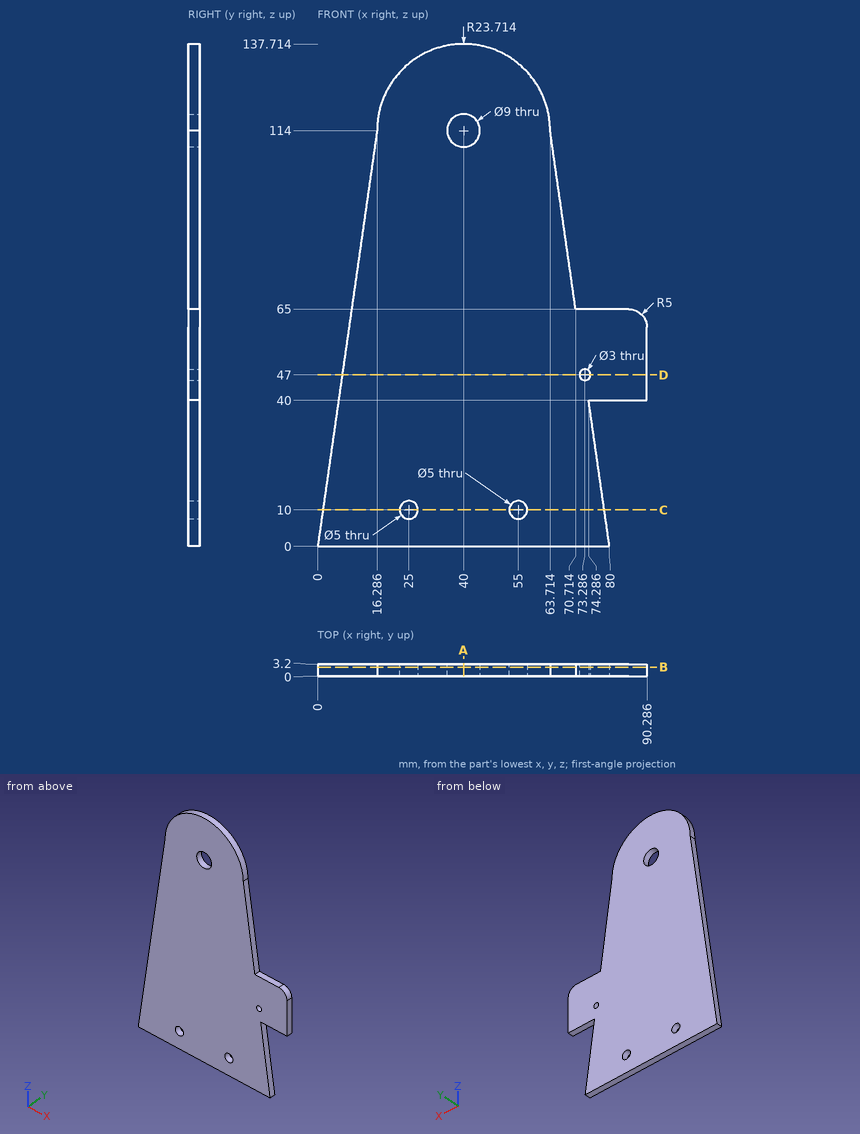
Can you work these out from the drawing? Everything is in mm from the part's minimum corner. Coordinates: 2 decimals unless noted, no trailing zeros. Loops run counter-clockwise (first coordinate to the right, second up) from the corner with the lowest first, then second, coordinate; pieces in that order, holes last.
1) I need wall thicknesses on probe 1 along Z at (x, y) = (40, 2.2); probe 2 along Z at (x, y) = (25, 1.2); probe 3 along X at (y, z) = (3, 116). Which ranges of each line are inside material? Lowest first, please.
2) Imagine slicing it at A-A on x = 40. List the corners of the cut face in (y, z) for me, plus the area to 3 significant figures.
3) For pin 1 (2.5 mm diameter, centred on x = 73.29, z = 47, fed in from -Y); pin 2 (1.6 mm diameter, centred on x = 81.5, y = 1, fed in from -Z); pin 3 (1.6 mm diameter, centred on x = 81, y = 1.5, fed in from +Z), each with a flat end and sliding along its axis, tell me the tip position at first contact or that it passes through.
4) Imagine slicing it at C-C on z = 10. List the corners of the cut face in (x, y) for me.
5) Imagine slicing it at D-D on z = 47. List the corners of the cut face in (x, y) for me, plus the area to 3 significant figures.
6) Imagine slicing it at B-B on y = 2.4. List the corners of the cut face in (x, z) for me, plus the area to 3 significant figures.
Completed:
1. probe 1: z = 0 to 109.5, 118.5 to 137.71
1. probe 2: z = 0 to 7.5, 12.5 to 132.37
1. probe 3: x = 16.37 to 35.97, 44.03 to 63.63
2. outline: (0, 0) - (3.2, 0) - (3.2, 109.5) - (0, 109.5) - close; (0, 118.5) - (3.2, 118.5) - (3.2, 137.71) - (0, 137.71) - close
2. area: 412 mm2
3. pin 1: passes through
3. pin 2: stops at z = 40
3. pin 3: stops at z = 65
4. outline: (1.43, 0) - (22.5, 0) - (22.5, 3.2) - (1.43, 3.2) - close; (27.5, 0) - (52.5, 0) - (52.5, 3.2) - (27.5, 3.2) - close; (57.5, 0) - (78.57, 0) - (78.57, 3.2) - (57.5, 3.2) - close
5. outline: (6.71, 0) - (71.79, 0) - (71.79, 3.2) - (6.71, 3.2) - close; (74.79, 0) - (90.29, 0) - (90.29, 3.2) - (74.79, 3.2) - close
5. area: 258 mm2
6. outline: (0, 0) - (80, 0) - (74.29, 40) - (90.29, 40) - (90.29, 60) arc R5 ccw to (85.29, 65) - (70.71, 65) - (63.71, 114) arc R23.71 ccw to (16.29, 114) - close; hole circle Ø5 at (25, 10); hole circle Ø9 at (40, 114); hole circle Ø5 at (55, 10); hole circle Ø3 at (73.29, 47)
6. area: 8,480 mm2
